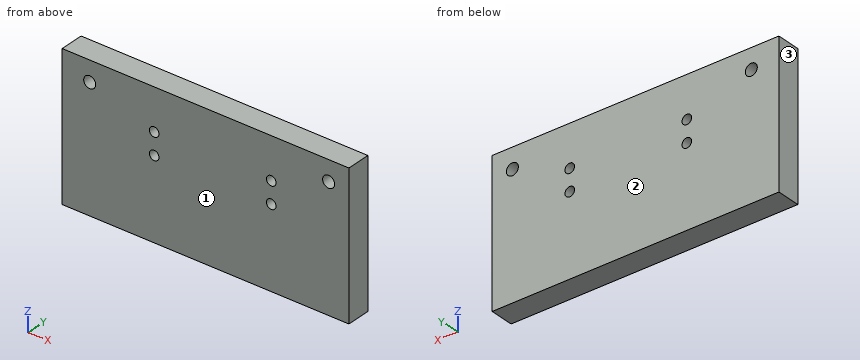
Autodesk Inventor part; units mm, degrees
ref_plane "YZ Plane" through (0, 0, 0) normal (1, 0, 0) x (0, 1, 0)
ref_plane "XZ Plane" through (0, 0, 0) normal (0, 1, 0) x (-1, 0, 0)
ref_plane "XY Plane" through (0, 0, 0) normal (0, 0, 1) x (1, 0, 0)
sketch "Sketch1" plane through (0, 0, 0) normal (0, 1, 0) x (-1, 0, 0)
  line L0 (54.4765, 8.5395) -> (-65.5235, 8.5395)
  line L1 (-65.5235, 8.5395) -> (-65.5235, -51.4605)
  line L2 (-65.5235, -51.4605) -> (54.4765, -51.4605)
  line L3 (54.4765, -51.4605) -> (54.4765, 8.5395)
  line L4 (42.9455, 0) -> (-57.0545, 0)
  circle A0 centre (42.9455, 0) radius 2.5
  circle A1 centre (-57.0545, 0) radius 2.5
  point P0 (0, 0)
  dimension "d0" = 120
  dimension "d1" = 60
  dimension "d2" = 100
  dimension "d3" = 5
  dimension "d4" = 5
extrude "Extrusion1" add sketch "Sketch1" along normal blind 10
sketch "Sketch2" plane through (0, 10, 0) normal (0, 1, 0) x (1, 0, 0)
  line L0 (-16.1382, 5.2435) -> (17.0718, 5.2435)
  circle A0 centre (-16.1382, 5.2435) radius 1
  circle A1 centre (17.0718, 5.2435) radius 1
  point P0 (0, 0)
  dimension "d7" = 33.21
  dimension "d8" = 2
  dimension "d9" = 2
extrude "Extrusion2" cut sketch "Sketch2" along normal blind 10
sketch "Sketch3" plane through (0, 10, 0) normal (0, 1, 0) x (1, 0, 0)
  point P0 (0, 0)
sketch "Sketch4" plane through (0, 10, 0) normal (0, 1, 0) x (1, 0, 0)
  circle A0 centre (-16.1382, 5.2435) radius 1
  circle A1 centre (30.8669, 5.2794) radius 1
  point P0 (0, 0)
  dimension "d13" = 2
extrude "Extrusion3" cut sketch "Sketch4" along normal blind 10 contours A1
sketch "Sketch5" plane through (0, 10, 0) normal (0, 1, 0) x (1, 0, 0)
  circle A0 centre (-16.1382, 5.2435) radius 1
  circle A1 centre (30.8669, 5.2794) radius 1
  circle A2 centre (30.8669, 14.2341) radius 2
  circle A3 centre (-16.1382, 14.2341) radius 2
  point P0 (0, 0)
  dimension "d20" = 4
  dimension "d21" = 4
extrude "Extrusion4" cut sketch "Sketch5" along normal blind 10 contours A2 | A3
sketch "Sketch6" plane through (0, 10, 0) normal (0, 1, 0) x (1, 0, 0)
  circle A0 centre (-15.9518, 8.8125) radius 2
  circle A1 centre (33.0446, 8.8125) radius 2
  circle A2 centre (-15.9518, 17.8231) radius 2
  circle A3 centre (33.0446, 17.8231) radius 2
  point P0 (0, 0)
  dimension "d24" = 4
  dimension "d26" = 4
  dimension "d30" = 4
extrude "Extrusion5" cut sketch "Sketch6" against normal blind 10
properties part number "servostand"
Geometry: final body of the model. Coordinates: model frame, mm. Face numbers are marked on the shaded views. Coordinates: 2 decimals unless noted, no trailing zeros. Loops run counter-clockwise (first coordinate to the right, second up) from the corner with the lowest first, then second, coordinate; pieces in that order, holes last. Notation, with made-up numbers: M 35,-15 L 63,-15 A10 cw 63,-1 Z; hole C 51,76 d10. An arc over 180 degrees is marked long. One line per item, written item: value. Start each with the question number.
1) Cut plane A-A (z = 0). Return loops of the section in (x, y), then the cut area to 3 significant figures.
2) Material intervals for L1, parallel to Z at x = 32, y = 7.75; L2, parallel to X at y = 3.5, z = -17; L3, parallel to Z at x = -15, y = 4.25, sorted ascending. Write a range as from..to.
3) Draft query along Y for the marked faces 1, 2 and 3. Return one class per face: released by +Y, released by -Y, zero draft, split by the parting line, or undercut.
Evaluation:
1. outline: M -54.48,0 L -45.45,0 L -45.45,10 L -54.48,10 Z; M -40.45,0 L 54.55,0 L 54.55,10 L -40.45,10 Z; M 59.55,0 L 65.52,0 L 65.52,10 L 59.55,10 Z
1. area: 1,100 mm^2
2. L1: -51.46..-19.53, -16.12..-10.52, -7.11..8.54
2. L2: -54.48..-17.77, -14.13..31.22, 34.87..65.52
2. L3: -51.46..-19.58, -16.06..-10.57, -7.05..8.54
3. face 1: released by -Y
3. face 2: released by +Y
3. face 3: zero draft
